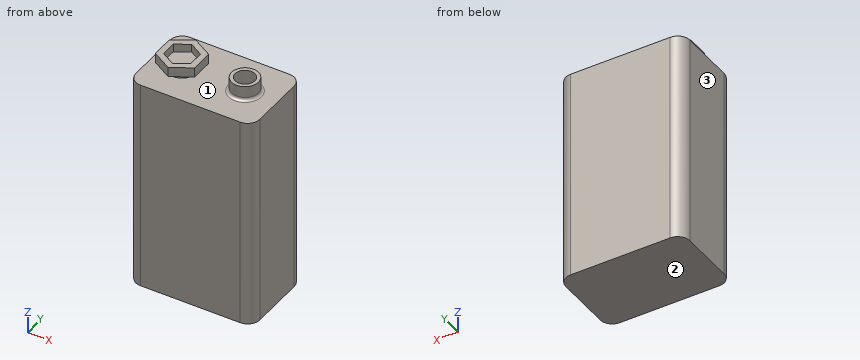
from build123d import *

# Parameters (mm, degrees)
SKETCH1_W           = 26.0604
SKETCH1_H           = 44.8564
BOSS_EXTRUDE1_DEPTH = 8.382
SKETCH2_R           = 2.8321
SKETCH2_R_2         = 2.0701
BOSS_EXTRUDE2_DEPTH = 3.2258
SKETCH3_R           = 3.1877
BOSS_EXTRUDE3_DEPTH = 1.016
BOSS_EXTRUDE4_DEPTH = 2.5654
FILLET1_R           = 2.54
FILLET2_R           = 0.635
BOSS_EXTRUDE5_DEPTH = 0.3175
FILLET3_R           = 0.635
SKETCH6_W           = 27.559321376
SKETCH6_H           = 27.598108844
CUT_EXTRUDE1_DEPTH  = 0.5334


with BuildPart() as part:
    # Sketch1 → Boss-Extrude1 (new, symmetric)
    with BuildSketch(Plane(origin=(0, 0, 0), x_dir=(1, 0, 0), z_dir=(0, 1, 0))):
        Rectangle(SKETCH1_W, SKETCH1_H)
    extrude(amount=BOSS_EXTRUDE1_DEPTH, both=True)

    # Sketch2 → Boss-Extrude2 (add)
    with BuildSketch(Plane.XY.offset(22.4282)):
        with Locations(Location((6.3119, 0, 0), (0, 0, 180))):
            Circle(SKETCH2_R)
        with Locations((6.3119, 0)):
            Circle(SKETCH2_R_2, mode=Mode.SUBTRACT)
    extrude(amount=BOSS_EXTRUDE2_DEPTH)

    # Sketch3 → Boss-Extrude3 (add)
    with BuildSketch(Plane.XY.offset(22.4282)):
        with Locations(Location((-6.9342, 0, 0), (0, 0, 180))):
            Circle(SKETCH3_R)
    extrude(amount=BOSS_EXTRUDE3_DEPTH)

    # Sketch4 → Boss-Extrude4 (add)
    with BuildSketch(Plane.XY.offset(23.4442)):
        Polygon((-2.8067, 2.383013236), (-6.9342, 4.766026472), (-11.0617, 2.383013236), (-11.0617, -2.383013236), (-6.9342, -4.766026472), (-2.8067, -2.383013236), align=None)
        Polygon((-9.7917, 1.649778394), (-9.7917, -1.649778394), (-6.9342, -3.299556788), (-4.0767, -1.649778394), (-4.0767, 1.649778394), (-6.9342, 3.299556788), align=None, mode=Mode.SUBTRACT)
    extrude(amount=BOSS_EXTRUDE4_DEPTH)

    # Fillet1
    fillet1_edges = [part.edges().sort_by_distance(p)[0] for p in [
        (-13.0302, 8.382, 0),
        (13.0302, 8.382, 0),
        (-13.0302, -8.382, 0),
        (13.0302, -8.382, 0),
    ]]
    fillet(fillet1_edges, radius=FILLET1_R)

    # Fillet2
    fillet2_edges = [part.edges().sort_by_distance(p)[0] for p in [
        (9.144, 0, 22.4282),
    ]]
    fillet(fillet2_edges, radius=FILLET2_R)

    # Sketch5 → Boss-Extrude5 (add)
    with BuildSketch(Plane.XY.offset(23.4442)):
        Polygon((-9.7917, -1.649778394), (-9.7917, 1.649778394), (-6.9342, 3.299556788), (-4.0767, 1.649778394), (-4.0767, -1.649778394), (-6.9342, -3.299556788), align=None)
    extrude(amount=BOSS_EXTRUDE5_DEPTH)

    # Fillet3
    fillet3_edges = [part.edges().sort_by_distance(p)[0] for p in [
        (-3.7465, 0, 23.4442),
    ]]
    fillet(fillet3_edges, radius=FILLET3_R)

    # Sketch6 → Cut-Extrude1 (cut)
    with BuildSketch(Plane.XY.offset(26.0096)):
        Rectangle(SKETCH6_W, SKETCH6_H)
    extrude(amount=-CUT_EXTRUDE1_DEPTH, mode=Mode.SUBTRACT)


solid = part.part
The model under review builds one solid part; all positions refer to its coordinate system, in mm. Face numbers are marked on the shaded views. Coordinates: 2 decimals unless noted, no trailing zeros. Loops run counter-clockwise (first coordinate to the right, second up) from the corner with the lowest first, then second, coordinate; pieces in that order, holes last. Notation, with made-up numbers: M -22.75,-18.75 L 16.25,-18.75 A20 cw 16.25,13.25 Z; hole C 5.25,1.5 d2. An arc over 180 degrees is marked long. Put each result on its own line as item: value. Start each with the question number.
Q1. Wall thickness on line 1 (Z direction, x = -4, y = 2.5); line 2 (Z direction, x = 11, y = 1.25); line 3 (Z direction, x = -5.25, y = -0.5): over which ranges is each line inside the solid? List them lowest first.
Q2. The part is to be moulded in two halves that separate along X. For the marked faces 1, 2 and 3, say which applies: +X half, -X half, draft (parallel to the pull), parting line (faces both ways), or undercut.
Q3. Add section B-B (y = 5.25). Write out the cut boundary in (x, z).
Q4. Clearance check with flat-ended pins moving along their axes: pin 1 (5 mm diameter, centred on x = 6.31, y = 0, fed in from +Z); pin 2 (1.4 mm diameter, centred on y = 0.5, z = 24.5, fed in from -X); pin 3 (1.6 mm diameter, centred on y = 0, z = 24, fed in from +X). State where each tip first meets the part, or that it passes through.
Answers:
1. line 1: z = -22.43 to 22.43, 23.44 to 25.48
1. line 2: z = -22.43 to 22.43
1. line 3: z = -22.43 to 23.76
2. face 1: undercut
2. face 2: draft
2. face 3: -X half
3. outline: M -13.03,-22.43 L 13.03,-22.43 L 13.03,22.43 L -13.03,22.43 Z
4. pin 1: stops at z = 25.48
4. pin 2: stops at x = -11.06
4. pin 3: stops at x = 9.14
